```python
from build123d import *

# Parameters (mm, degrees)
F0_W     = 208.457162
F0_H     = 14.880452
F0_R     = 0.762
F0_W_2   = 187.614396
F0_H_2   = 3.722524
F1_DEPTH = 9.525
F2_DEPTH = 8.89


with BuildPart() as f1:
    # F0 (on Front) → F1 (new body, symmetric)
    with BuildSketch(Plane.XZ):
        Rectangle(F0_W, F0_H)
        with Locations((-99.507612, 0)):
            Circle(F0_R, mode=Mode.SUBTRACT)
        Rectangle(F0_W_2, F0_H_2, mode=Mode.SUBTRACT)
        with Locations((99.507612, 0)):
            Circle(F0_R, mode=Mode.SUBTRACT)
        Rectangle(F0_W_2, F0_H_2)
    extrude(amount=F1_DEPTH, both=True)

    # F0 (on Front) → F2 (cut, symmetric)
    with BuildSketch(Plane.XZ):
        Rectangle(F0_W, F0_H)
        with Locations((-99.507612, 0)):
            Circle(F0_R, mode=Mode.SUBTRACT)
        Rectangle(F0_W_2, F0_H_2, mode=Mode.SUBTRACT)
        with Locations((99.507612, 0)):
            Circle(F0_R, mode=Mode.SUBTRACT)
    extrude(amount=F2_DEPTH, both=True, mode=Mode.SUBTRACT)


solid = f1.part
```
Read the model definition and answer for the solid it produces. Units are mm, in the model's axes. A direction names the side the tool comes from. Give positions to 0.01 mm unless a question says otherwise; leave off trailing zeros. Loops run counter-clockwise (first coordinate to the right, second up) from the corner with the lowest first, then second, coordinate; pieces in that order, holes last.
Item 1: Each of these flat-tipped pins is pushed along its axis until it touches: pin 1 Ø5 at (y, z) = (-6, 4) entering from -X; pin 2 Ø6 at (x, y) = (5, 6.5) entering from -Z; pin 3 Ø4 at (x, y) = (30, -2.5) entering from -Z; pin 4 Ø3 at (y, z) = (5.5, -6) entering from -X. Where does it stop, or does it pass through?
Item 2: Find the intervals of material crossed by line 1 along Y through (x, z) = (59.5, -5.25) (3 decimals); line 2 along Z through (x, y) = (-51.5, -7.25); line 3 along X through (y, z) = (8.25, -0.5), in increasing order.
Item 3: The part is cut by section A-A (z = -4.5). Write down the section's boundary in (x, y) (3 decimals).
Item 4: The mould has two halves that part along Y. Classify faces 1 (the flat face through (-1, 9.525, 0)), 2 (the flat face through (-1, -9.525, 0)), 3 (the flat face through (-1, 0, 1.861)): released by +Y, released by -Y, zero draft, split by the parting line, or undercut.
Item 5: The part is cut by section B-B (x = -86). Write down the section's boundary in (y, z) (3 decimals).
Item 6: For faces 4 (the flat face through (93.807, 0, 0)), 5 (the flat face through (-93.807, 0, 0)), 6 (the flat face through (-1, 0, -1.861)), determine the directions among +Z, -Z, +X, -X, +Y, -Y from which every point of the face is accessible in a straight line to the end or side of a thin tool.
Item 7: The part is cut by section C-C (y = 0.25). Write down the section's boundary in (x, z), and give its area (3 significant figures).
Taken from the geometry:
1. pin 1: stops at x = -93.81
1. pin 2: stops at z = -7.44
1. pin 3: stops at z = -1.86
1. pin 4: passes through
2. line 1: y = -9.525 to -8.89, 8.89 to 9.525
2. line 2: z = -1.86 to 1.86
2. line 3: x = -93.81 to 93.81
3. outline: (-104.229, -9.525) - (104.229, -9.525) - (104.229, -8.89) - (-104.229, -8.89) - close; (-104.229, 8.89) - (104.229, 8.89) - (104.229, 9.525) - (-104.229, 9.525) - close
4. face 1: released by +Y
4. face 2: released by -Y
4. face 3: undercut
5. outline: (-9.525, -7.44) - (-8.89, -7.44) - (-8.89, -1.861) - (8.89, -1.861) - (8.89, -7.44) - (9.525, -7.44) - (9.525, 7.44) - (8.89, 7.44) - (8.89, 1.861) - (-8.89, 1.861) - (-8.89, 7.44) - (-9.525, 7.44) - close
6. face 4: +Z, -Z, +X
6. face 5: +Z, -Z, -X
6. face 6: -Z, +X, -X
7. outline: (-93.81, -1.86) - (93.81, -1.86) - (93.81, 1.86) - (-93.81, 1.86) - close
7. area: 698 mm2
